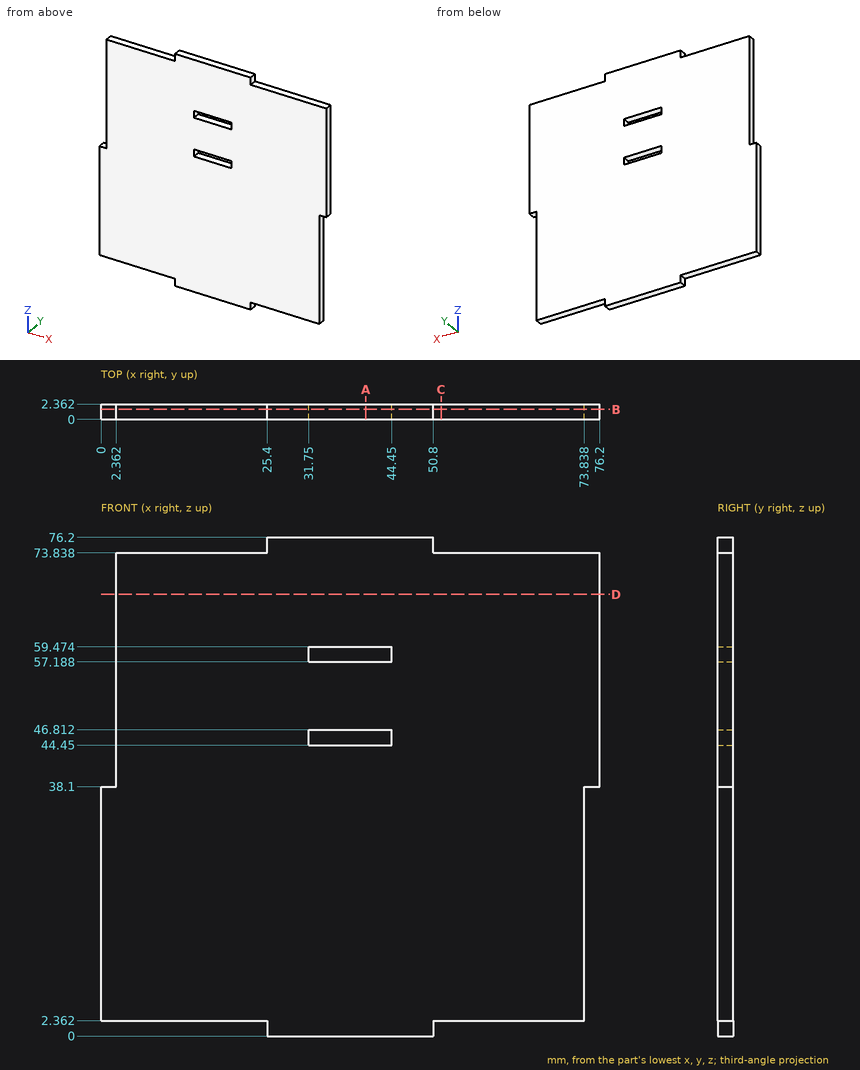
Source: three-view drawing plus pictorial views. Frame: mm from the lowest corner of the part. Round coordinates to 2 decimals unless told otherwise and drop trailing zeros. Loops run counter-clockwise (first coordinate to the right, second up) from the corner with the lowest first, then second, coordinate; pieces in that order, holes last. Notation, with made-up numbers: M 16,-14 L 38,-14 A23 ccw 38,2 Z; hole C 18,-13 d4. An arc over 180 degrees is marked long. Put each result on its own line as item: value.
(1) Section C-C, the plane x = 52. Return loops of the section in (y, z).
Solutions:
outline: M 0,2.36 L 2.36,2.36 L 2.36,73.84 L 0,73.84 Z
(2) Section D-D, the plane z = 67.5. Return loops of the section in (x, y), and give its area (3 significant figures).
Solutions:
outline: M 2.36,0 L 76.2,0 L 76.2,2.36 L 2.36,2.36 Z
area: 174 mm²
(3) First-contact query: pin 1 (1.2 mm diameter, centred on x = 1.5, y = 1.5, fed in from +Z); pin 2 (1.2 mm diameter, centred on y = 1.5, z = 23, fed in from +X); pin 3 (0.7 mm diameter, centred on x = 9.5, y = 0.5, fed in from -Z). Flat tips, straight axial feed; report the tip coordinate or a pass-through.
Solutions:
pin 1: z = 38.1
pin 2: x = 73.84
pin 3: z = 2.36
(4) Section B-B, the plane y = 1.55. Return loops of the section in (x, z).
Solutions:
outline: M 0,2.36 L 25.4,2.36 L 25.4,0 L 50.8,0 L 50.8,2.36 L 73.84,2.36 L 73.84,38.1 L 76.2,38.1 L 76.2,73.84 L 50.8,73.84 L 50.8,76.2 L 25.4,76.2 L 25.4,73.84 L 2.36,73.84 L 2.36,38.1 L 0,38.1 Z; hole M 31.75,44.45 L 44.45,44.45 L 44.45,46.81 L 31.75,46.81 Z; hole M 31.75,57.19 L 44.45,57.19 L 44.45,59.47 L 31.75,59.47 Z
(5) Section A-A, the plane x = 40.5. Return loops of the section in (y, z), and give its area (3 significant figures).
Solutions:
outline: M 0,0 L 2.36,0 L 2.36,44.45 L 0,44.45 Z; M 0,46.81 L 2.36,46.81 L 2.36,57.19 L 0,57.19 Z; M 0,59.47 L 2.36,59.47 L 2.36,76.2 L 0,76.2 Z
area: 169 mm²
(6) Ray query, line 1 (Z direction, x = 44, y = 0.8); line 2 (X direction, y = 0.6, z = 59); line 3 (X direction, y = 0.25, z = 31.5). Return the intervals inside material, ascending. Write a range as [from, to].
Solutions:
line 1: [0, 44.45], [46.81, 57.19], [59.47, 76.2]
line 2: [2.36, 31.75], [44.45, 76.2]
line 3: [0, 73.84]
